Autodesk Inventor part; units mm, degrees
ref_plane "YZ Plane" through (0, 0, 0) normal (1, 0, 0) x (0, 1, 0)
ref_plane "XZ Plane" through (0, 0, 0) normal (0, 1, 0) x (-1, 0, 0)
ref_plane "XY Plane" through (0, 0, 0) normal (0, 0, 1) x (1, 0, 0)
sketch "Sketch1" plane through (0, 0, 0) normal (0, 1, 0) x (-1, 0, 0)
  circle A0 centre (0, 0) radius 2
  dimension "d0" = 4
extrude "Extrusion1" add sketch "Sketch1" against normal blind 28
sketch "Sketch2" plane through (0, -28, 0) normal (0, -1, 0) x (1, 0, 0)
  circle A0 centre (0, 0) radius 2
  line L0 (-1.3229, 1.5) -> (1.3229, 1.5)
  circle A1 centre (0, 0) radius 2
  dimension "d3" = 0.5
extrude "Extrusion2" cut sketch "Sketch2" against normal through all contours L0 A0 picked at (-0.3089, 1.5908)
chamfer "Chamfer1" distance 0.2 angle 45 4 edges at (0, -28, -2) (0, -28, 1.5) (0, 0, -2) (0, 0, 1.5)
properties part number "10-0028" material "Aluminum 6061"
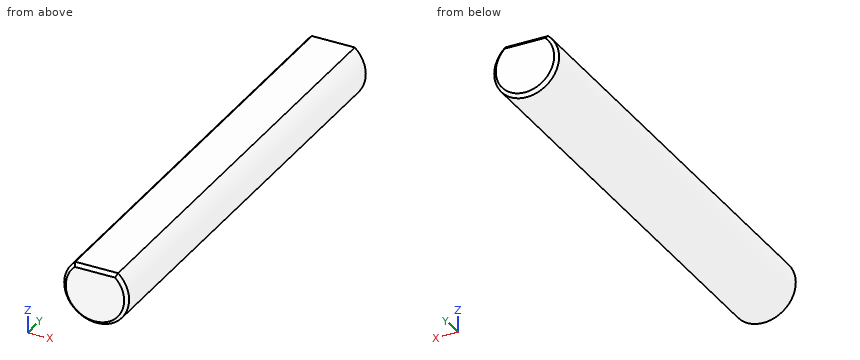
For this review, take the finished solid that the model builds, in its own axes (mm). Coordinates: 2 decimals unless noted, no trailing zeros. Write each loop counter-clockwise with the first axis right and the second up, starting at its lowest first coordinate (ties: lowest second). Pieces come first, ordered by that corner, then holes. Notation, with made-up numbers: (86, 65.25) - (96, 65.25) arc R21 cw to (96, 79.25) - close; hole circle Ø6 at (30, -2). An arc over 180 degrees is marked (long way). Answer in a Markdown table with one row per item. Add a question column.
Q1. We need section A-A, the plane y = -6.25. State the section outline as (x, z) points, and give its area (3 significant figures).
Q2. For probe 1 along Z at (x, y) = (-1.5, -8.5); probe 2 along X at (y, z) = (-26.25, 0.1); probe 3 along X at (y, z) = (-4.5, -1.65), list the stretches that pass through material, from the lowest coordinate up.
Q3. For P1, Ø1.5, axis at y = -3, z = 1, coming from the +X side, flat-tipped, find the tip position at first contact; note if it passes through.
Answer list:
| question | item | result |
|---|---|---|
| 1 | outline | (-1.32, 1.5) arc R2 ccw (long way) to (1.32, 1.5) - close |
| 1 | area | 11.7 mm2 |
| 2 | probe 1 | z = -1.32 to 1.32 |
| 2 | probe 2 | x = -2 to 2 |
| 2 | probe 3 | x = -1.13 to 1.13 |
| 3 | P1 | stops at x = 1.98 |
